Check sheet for the drawn part. Datum: minimum x, y, z corner. Units: mm. Coordinates: 2 decimals unless noted, no trailing zeros. Write each loop counter-clockwise with the first axis right and the second up, starting at its lowest first coordinate (ties: lowest second). Pieces come first, ordered by that corner, then holes. Notation, with made-up numbers: (73.5, -31) -> (88.5, -31) arc R20 ccw to (88.5, -15) -> close; hole circle Ø11 at (1.25, 9). An arc over 180 degrees is marked (long way). One line per question, with ' | ' between items.
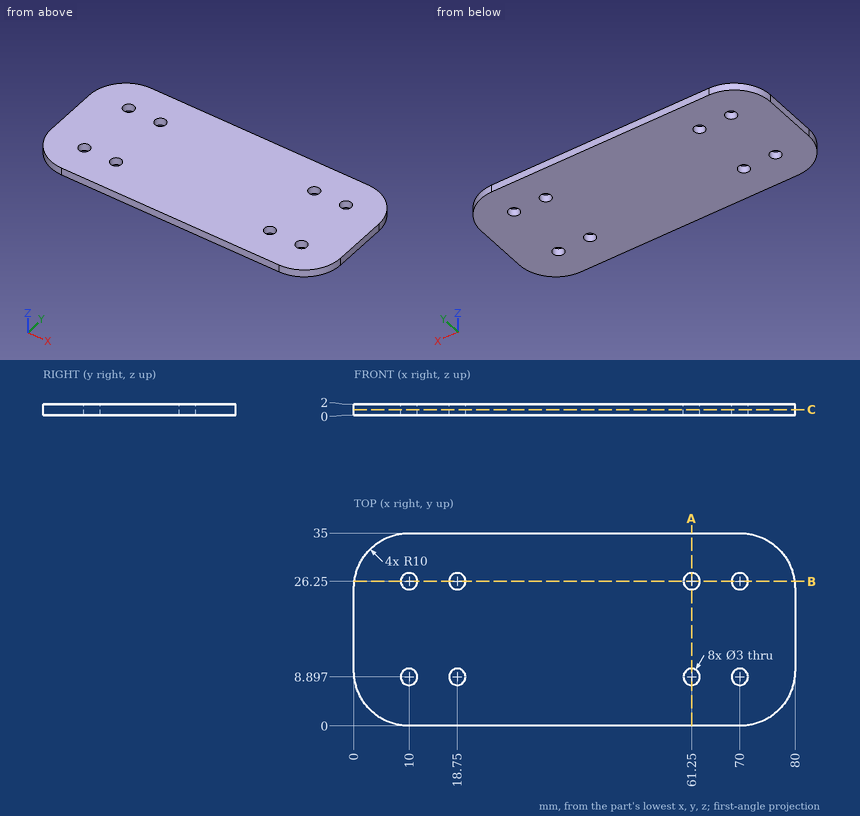
1. Cross-section at B-B on y = 26.25. Record the boundary of the cut face in (x, z), and give its area (3 significant figures).
Worked answers:
outline: (0.08, 0) -> (8.5, 0) -> (8.5, 2) -> (0.08, 2) -> close; (11.5, 0) -> (17.25, 0) -> (17.25, 2) -> (11.5, 2) -> close; (20.25, 0) -> (59.75, 0) -> (59.75, 2) -> (20.25, 2) -> close; (62.75, 0) -> (68.5, 0) -> (68.5, 2) -> (62.75, 2) -> close; (71.5, 0) -> (79.92, 0) -> (79.92, 2) -> (71.5, 2) -> close | area: 136 mm²
2. Go/stop test with a flat-tipped pin: P1, Ø2.5, axis at x = 61.25, y = 26.25, coming from the +Z side. Record where the tip stops, or that it passes through.
Worked answers:
P1: through
3. Cross-section at C-C on z = 1. Give the number of separate pieces and of enclosed holes in the cut face, and give its area (3 significant figures).
Worked answers:
separate pieces: 1 | enclosed holes: 8 | area: 2,660 mm²
4. Cross-section at A-A on x = 61.25. Record the boundary of the cut face in (y, z).
Worked answers:
outline: (0, 0) -> (7.4, 0) -> (7.4, 2) -> (0, 2) -> close; (10.4, 0) -> (24.75, 0) -> (24.75, 2) -> (10.4, 2) -> close; (27.75, 0) -> (35, 0) -> (35, 2) -> (27.75, 2) -> close
5. Material ranges on line 1 (Y direction, x = 61.25, z = 1); line 2 (X direction, y = 9, z = 0.2); line 3 (X direction, y = 27, z = 1.6), recorded low to high. Write a range as from..to.
Worked answers:
line 1: 0..7.4, 10.4..24.75, 27.75..35 | line 2: 0.05..8.5, 11.5..17.25, 20.25..59.75, 62.75..68.5, 71.5..79.95 | line 3: 0.2..8.7, 11.3..17.45, 20.05..59.95, 62.55..68.7, 71.3..79.8
